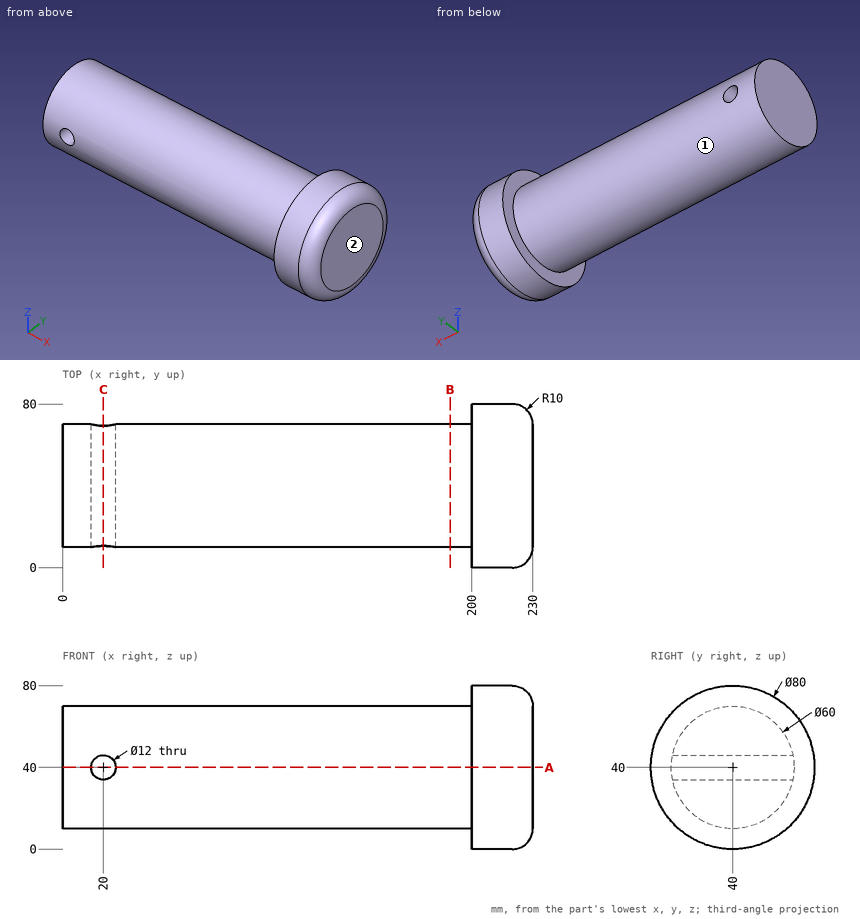
Print and shaded views of the part. All mm, measured from the part's lowest x, y and z. A direction names the side the tool comes from. Give positions to 0.01 mm unless a question says otherwise; leave off trailing zeros. Write each loop counter-clockwise with the first axis right and the second up, starting at its lowest first coordinate (ties: lowest second). Pieces come first, ordered by that corner, then holes. Notation, with made-up numbers: (27.25, 18.5) - (70.25, 18.5) arc R26 ccw to (70.25, 40.5) - close; hole circle Ø4 at (71, 39.25). An arc over 180 degrees is marked (long way). Put each result on its own line as item: value.
(1) Saw through at B-B (x = 189.5). List the corners of the cut face in (y, z), then the cut area to 3 significant figures.
Working result:
outline: circle Ø60 at (40, 40)
area: 2,830 mm^2
(2) Drop flat-ended pins along their axis: pin 1 Ø1 at (x, y) = (142, 19.5) entering from +Z; pin 2 Ø2 at (x, z) = (196, 46) entering from -Y; pin 3 Ø5 at (x, z) = (65, 30) entering from -Y. Give the stop position or say it passes through.
Working result:
pin 1: z = 62.36
pin 2: y = 10.42
pin 3: y = 10.95
(3) Tool access for the marked faces 1 and 2: list every direction of +Z, -Z, +X, -X, +Y, -Y with a clear straight run to the whole face (end or side of a thin tool).
Working result:
face 1: -X
face 2: +Z, -Z, +X, +Y, -Y
(4) Saw through at C-C (x = 20). List the corners of the cut face in (y, z), then the cut area to 3 significant figures.
Working result:
outline: (10.61, 34) arc R30 ccw to (69.39, 34) - close; (10.61, 46) - (69.39, 46) arc R30 ccw to start
area: 2,110 mm^2
(5) Wall check: L1, parallel to X at y = 39, z = 40; L2, parallel to Z at x = 20, y = 54; L3, parallel to Z at x = 20, y = 35. Give the ranges that are in metal, low to high.
Working result:
L1: 0 to 14, 26 to 230
L2: 13.47 to 34, 46 to 66.53
L3: 10.42 to 34, 46 to 69.58
(6) Saw through at A-A (z = 40). List the corners of the cut face in (x, y), then the cut area to 3 significant figures.
Working result:
outline: (0, 10) - (14, 10) - (14, 70) - (0, 70) - close; (26, 10) - (200, 10) - (200, 0) - (220, 0) arc R10 ccw to (230, 10) - (230, 70) arc R10 ccw to (220, 80) - (200, 80) - (200, 70) - (26, 70) - close
area: 13,600 mm^2
